Geometry check sheet. Reference: the model listing, model coordinates, mm. Face numbers are marked on the shaded views. A direction names the side the tool comes from. Give positions to 0.01 mm unless a question says otherwise; leave off trailing zeros. Order: outer loops, then holes, each group sorted by start corner. A loop starts at its lowest first (then second) coordinate and runs counter-clockwise, first axis right, second up. Notation, with made-up numbers: (82.5, 86.25) - (119.5, 86.25) arc R29 cw to (119.5, 122.25) - close; hole circle Ø11 at (68.5, 51). An arc over 180 degrees is marked (long way). Put each result on its own line as item: value. Start each with the question number.
```python
from build123d import *

# Parameters (mm, degrees)
SKETCH2_W                                           = 200
SKETCH2_H                                           = 300
BOSS_EXTRUDE1_DEPTH                                 = 150
SHELL1_T                                            = -2
SKETCH4_W                                           = 20
SKETCH4_H                                           = 15
SKETCH4_W_2                                         = 15
SKETCH4_H_2                                         = 20
BOSS_EXTRUDE2_DEPTH                                 = 2
CSK_FOR_M2_COUNTERSUNK_FLAT_HEAD_SCREW1_D           = 2.4
CSK_FOR_M2_COUNTERSUNK_FLAT_HEAD_SCREW1_DEPTH       = 30
CSK_FOR_M2_COUNTERSUNK_FLAT_HEAD_SCREW1_CSINK_D     = 4.4
CSK_FOR_M2_COUNTERSUNK_FLAT_HEAD_SCREW1_CSINK_ANGLE = 90
CSK_FOR_M2_COUNTERSUNK_FLAT_HEAD_SCREW1_TIP         = 0.721032743
SKETCH6_W                                           = 200
SKETCH6_H                                           = 1
EXTRUDE_THIN1_DEPTH                                 = 296
CUT_EXTRUDE1_DEPTH                                  = 2
F_3_0MM_DOWEL_HOLE1_D                               = 3
F_3_0MM_DOWEL_HOLE1_DEPTH                           = 30
F_3_0MM_DOWEL_HOLE1_TIP                             = 0.901290929


with BuildPart() as part:
    # Sketch2 → Boss-Extrude1 (new body)
    with BuildSketch(Plane(origin=(0, 0, 0), x_dir=(1, 0, 0), z_dir=(0, 1, 0))):
        Rectangle(SKETCH2_W, SKETCH2_H)
    extrude(amount=BOSS_EXTRUDE1_DEPTH)

    # Shell1
    shell1_openings = [part.faces().sort_by_distance(p)[0] for p in [
        (0, 150, 0),
    ]]
    offset(amount=SHELL1_T, openings=shell1_openings, kind=Kind.INTERSECTION)

    # Sketch4 → Boss-Extrude2 (add)
    with BuildSketch(Plane(origin=(0, 0, 0), x_dir=(1, 0, 0), z_dir=(0, 1, 0))):
        with Locations((-90, -157.5)):
            Rectangle(SKETCH4_W, SKETCH4_H)
        with Locations((90, -157.5)):
            Rectangle(SKETCH4_W, SKETCH4_H)
        with Locations((107.5, 140)):
            Rectangle(SKETCH4_W_2, SKETCH4_H_2)
        with Locations((107.5, -115)):
            Rectangle(SKETCH4_W_2, SKETCH4_H_2)
    extrude(amount=BOSS_EXTRUDE2_DEPTH)

    # CSK for M2 Countersunk Flat Head Screw1
    with Locations(Plane(origin=(107.5, 2, -140), x_dir=(0, 0, 1), z_dir=(0, 1, 0))):
        with Locations((0, 0), (255, 0), (297.5, -17.5), (297.5, -197.5)):
            CounterSinkHole(CSK_FOR_M2_COUNTERSUNK_FLAT_HEAD_SCREW1_D / 2, CSK_FOR_M2_COUNTERSUNK_FLAT_HEAD_SCREW1_CSINK_D / 2, depth=CSK_FOR_M2_COUNTERSUNK_FLAT_HEAD_SCREW1_DEPTH, counter_sink_angle=CSK_FOR_M2_COUNTERSUNK_FLAT_HEAD_SCREW1_CSINK_ANGLE)
            with Locations((0, 0, -(CSK_FOR_M2_COUNTERSUNK_FLAT_HEAD_SCREW1_DEPTH + CSK_FOR_M2_COUNTERSUNK_FLAT_HEAD_SCREW1_TIP / 2))):  # 118° drill point
                Cone(0, CSK_FOR_M2_COUNTERSUNK_FLAT_HEAD_SCREW1_D / 2, CSK_FOR_M2_COUNTERSUNK_FLAT_HEAD_SCREW1_TIP, mode=Mode.SUBTRACT)

    # Sketch6 → Extrude-Thin1 (add)
    with BuildSketch(Plane(origin=(0, 0, 148), x_dir=(-1, 0, 0), z_dir=(0, 0, -1))):
        with Locations((0, 44.5)):
            Rectangle(SKETCH6_W, SKETCH6_H)
        with Locations((0, 89.5)):
            Rectangle(SKETCH6_W, SKETCH6_H)
        with Locations((0, 134.5)):
            Rectangle(SKETCH6_W, SKETCH6_H)
    extrude(amount=EXTRUDE_THIN1_DEPTH)

    # Sketch7 → Cut-Extrude1 (cut)
    with BuildSketch(Plane.ZY.offset(100)):
        Polygon((-150, 0), (165, 0), (165, 2), (150, 2), (150, 150), (-150, 150), align=None)
    extrude(amount=-CUT_EXTRUDE1_DEPTH, mode=Mode.SUBTRACT)

    # Ø3.0mm Dowel Hole1
    with Locations(Plane(origin=(0, 135, 0), x_dir=(1, 0, 0), z_dir=(0, 1, 0))):
        with Locations((0, 0), (80, 140), (0, 140), (80, 0)):
            Hole(F_3_0MM_DOWEL_HOLE1_D / 2, depth=F_3_0MM_DOWEL_HOLE1_DEPTH)
            with Locations((0, 0, -(F_3_0MM_DOWEL_HOLE1_DEPTH + F_3_0MM_DOWEL_HOLE1_TIP / 2))):  # 118° drill point
                Cone(0, F_3_0MM_DOWEL_HOLE1_D / 2, F_3_0MM_DOWEL_HOLE1_TIP, mode=Mode.SUBTRACT)


solid = part.part
```
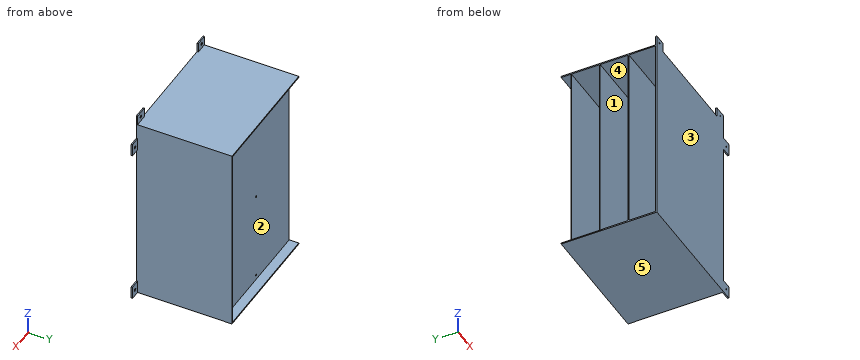
Item 1: Gauge pin test, flat ends, axial feed: pin 1 Ø2 at (y, z) = (87.5, 52.5) entering from +X; pin 2 Ø12 at (x, y) = (42.5, 144.5) entering from +Z; pin 3 Ø12 at (x, z) = (-32.5, -87.5) entering from +Y. Record the tip position at first contact, or that the pin passes through.
Item 2: Thickness scan on line 1 along Y through (x, z) = (11.5, -67.5); line 2 along Z through (x, y) = (107.5, 0.35); line 3 along X through (y, z) = (134.2, -140). Record the ranges inside material, lowest first.
Item 3: Cross-section at B-B (z = 11.5). Enter the section's corners in (x, y), and give its area (3 significant figures).
Item 4: Cross-section at C-C (y = 107). Enter the section's corners in (x, z), and give its area (3 significant figures).
Item 5: Set-up check for the marked faces 1 and 2: record each of +Z, -Z, +X, -X, +Y, -Y from which the full face is reachable in a straight line by a thin tool's end or side.
Item 6: Release check for a two-part mould opening along Z. For the marked faces 3, 4 and 5 record: +Z half, -Z half, draft (parallel to the pull), parting line (faces both ways), or undercut.
Item 7: Cross-section at A-A (x = 8.5). Enter the section's corners in (y, z), and give its area (3 significant figures).
Recorded:
1. pin 1: stops at x = 100
1. pin 2: stops at z = 150
1. pin 3: stops at y = 135
2. line 1: y = 0 to 2, 44 to 45, 89 to 90, 134 to 135
2. line 2: z = -150 to -141.2, -138.8 to -130, 105 to 113.8, 116.2 to 125
2. line 3: x = -98 to -1.5, 1.5 to 78.5, 81.5 to 100
3. outline: (-98, 0) - (100, 0) - (100, 150) - (98, 150) - (98, 135) - (-98, 135) - (-98, 134) - (98, 134) - (98, 90) - (-98, 90) - (-98, 89) - (98, 89) - (98, 45) - (-98, 45) - (-98, 44) - (98, 44) - (98, 2) - (-98, 2) - close
3. area: 1,280 mm^2
4. outline: (-98, -150) - (100, -150) - (100, 150) - (-98, 150) - (-98, 148) - (98, 148) - (98, -148) - (-98, -148) - close
4. area: 1,380 mm^2
5. face 1: -X
5. face 2: -X, +Y
6. face 3: draft
6. face 4: undercut
6. face 5: -Z half
7. outline: (0, -150) - (150, -150) - (150, -148) - (135, -148) - (135, 148) - (150, 148) - (150, 150) - (0, 150) - close; hole (2, -148) - (44, -148) - (44, 148) - (2, 148) - close; hole (45, -148) - (89, -148) - (89, 148) - (45, 148) - close; hole (90, -148) - (134, -148) - (134, 148) - (90, 148) - close
7. area: 2,080 mm^2
